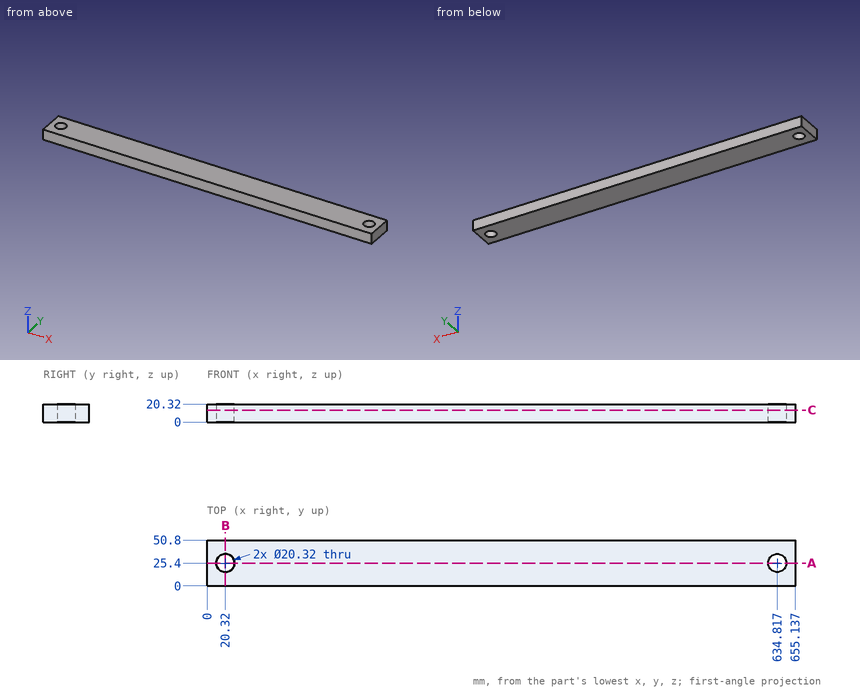
Source: three-view drawing plus pictorial views. Frame: mm from the lowest corner of the part. Round coordinates to 2 decimals unless told otherwise and drop trailing zeros. Write each loop counter-clockwise with the first axis right and the second up, starting at its lowest first coordinate (ties: lowest second). Pieces come first, ordered by that corner, then holes. Notation, with made-up numbers: M -15,18.5 L -10,18.5 A28 cw -10,56.5 Z; hole C 43,82 d1. An arc over 180 degrees is marked long. One line per item, written item: value. Start each with the question number.
Item 1: Section query B-B (x = 20.32). Return the cut outline in (y, z), plus the area to 3 significant figures.
Item 2: Section query C-C (z = 13.5). Return the cut outline in (x, y).
Item 3: Section query A-A (y = 25.4). Return the cut outline in (x, z).
Item 4: Ray query, L1, parallel to X at y = 26.5, z = 10.25; L2, parallel to X at y = 21.5, z = 13; L3, parallel to Y at x = 20.32, z = 6.75. Return the intervals inside material, ascending. Write a range as from..to.
Result set:
1. outline: M 0,0 L 15.24,0 L 15.24,20.32 L 0,20.32 Z; M 35.56,0 L 50.8,0 L 50.8,20.32 L 35.56,20.32 Z
1. area: 619 mm²
2. outline: M 0,0 L 655.14,0 L 655.14,50.8 L 0,50.8 Z; hole C 20.32,25.4 d20.32; hole C 634.82,25.4 d20.32
3. outline: M 0,0 L 10.16,0 L 10.16,20.32 L 0,20.32 Z; M 30.48,0 L 624.66,0 L 624.66,20.32 L 30.48,20.32 Z; M 644.98,0 L 655.14,0 L 655.14,20.32 L 644.98,20.32 Z
4. L1: x = 0..10.22, 30.42..624.72, 644.92..655.14
4. L2: x = 0..10.94, 29.7..625.44, 644.2..655.14
4. L3: y = 0..15.24, 35.56..50.8
